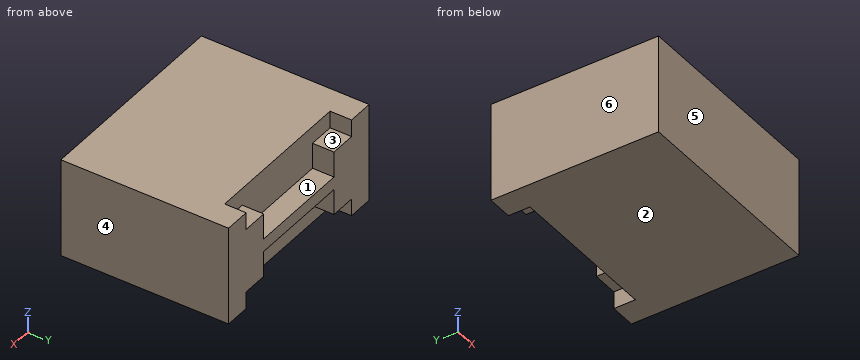
from build123d import *

# Parameters (mm, degrees)
SKETCH_1_W               = 240
SKETCH_1_H               = 195
EXTRUDE_1_DEPTH          = 57.5
CUT_EXTRUDE_1_DEPTH      = 165.962116863
CUT_EXTRUDE_1_DEPTH_BACK = 50
CUT_EXTRUDE_START        = -20
CUT_EXTRUDE_2_OUTLINE_W  = 30
CUT_EXTRUDE_2_OUTLINE_H  = 25
CUT_EXTRUDE_2_DEPTH      = 20


# Read off the part's stored shape, not the designer's step: 切除-拉伸2
with BuildPart() as part:
    # 草图1 → 凸台-拉伸1 (new body)
    with BuildSketch(Plane.XY):
        Rectangle(SKETCH_1_W, SKETCH_1_H)
    extrude(amount=EXTRUDE_1_DEPTH)

    # 草图2 → 切除-拉伸1 (cut, two sides: drawn at the far end of the back side and taken through both)
    with BuildSketch(Plane.XY.offset(57.5).offset(-CUT_EXTRUDE_1_DEPTH_BACK)):
        Polygon((-60, 638.254180389), (-60, 97.5), (-60, 72.5), (60, 72.5), (60, 97.5), (60, 638.254180389), (60, 1719.762541166), (-60, 1719.762541166), align=None)
    extrude(amount=CUT_EXTRUDE_1_DEPTH + CUT_EXTRUDE_1_DEPTH_BACK, mode=Mode.SUBTRACT)

    # 切除-拉伸2 outline → 切除-拉伸2 (cut)
    with BuildSketch(Plane.XY.offset(57.5).offset(CUT_EXTRUDE_START)):
        with Locations((-75, 85)):
            Rectangle(CUT_EXTRUDE_2_OUTLINE_W, CUT_EXTRUDE_2_OUTLINE_H)
    cut_extrude_2 = extrude(amount=CUT_EXTRUDE_2_DEPTH, mode=Mode.SUBTRACT)

    # 镜向1: 切除-拉伸2 across plane
    add(cut_extrude_2.mirror(Plane(origin=(0, 0, 0), x_dir=(0, 0, 1), z_dir=(1, 0, 0))), mode=Mode.SUBTRACT)

    # 镜向2: part across plane


with BuildPart() as part_1:
    add(part.part)
    add(part.part.mirror(Plane(origin=(0, 0, 0), x_dir=(1, 0, 0), z_dir=(0, 0, -1))))


solid = part_1.part
Geometry check sheet. Reference: the model listing, model coordinates, mm. Face numbers are marked on the shaded views. A direction names the side the tool comes from. Round coordinates to 2 decimals unless told otherwise and drop trailing zeros. Write each loop counter-clockwise with the first axis right and the second up, starting at its lowest first coordinate (ties: lowest second). Pieces come first, ordered by that corner, then holes.
Item 1: Mould release check, pull along X, two halves, no side actions. Record for the marked faces 3, 4, 5 and 6: +X half, -X half, draft (parallel to the pull), parting line (faces both ways), or undercut.
Determined:
face 3: undercut
face 4: +X half
face 5: draft
face 6: -X half
Item 2: Access from +Z, -Z, +X, -X, +Y, -Y to the whole of each face (thin tool, end or side, straight path). Record for the marked faces 1 and 2.
Determined:
face 1: +Z, +Y
face 2: -Z, +X, -X, +Y, -Y
Item 3: Section check A-A (z = 16.5). Record the boundary of the cut face in (x, y), plus the area to 3 significant figures.
Determined:
outline: (-120, -97.5) - (120, -97.5) - (120, 97.5) - (60, 97.5) - (60, 72.5) - (-60, 72.5) - (-60, 97.5) - (-120, 97.5) - close
area: 43,800 mm2
Item 4: Material ranges on line 1 along X through (y, z) = (85, -28); line 2 along Y through (x, z) = (63.5, -48); line 3 along Z through (x, y) = (37.5, 87), recorded low to high.
Determined:
line 1: x = -120 to -60, 60 to 120
line 2: y = -97.5 to 72.5
line 3: z = -7.5 to 7.5
Item 5: Go/stop test with flat-tipped pins: pin 1 Ø15 at (x, z) = (-43, 40.5) entering from +Y; pin 2 Ø7.5 at (x, y) = (69.5, 91) entering from +Z; pin 3 Ø7.5 at (x, y) = (1.5, 82) entering from +Z; pin 4 Ø4 at (x, z) = (54.5, -9) entering from +Y. Record where each tip stops, or that it passes through.
Determined:
pin 1: stops at y = 72.5
pin 2: stops at z = 37.5
pin 3: stops at z = 7.5
pin 4: stops at y = 97.5
Item 6: Section check B-B (x = 66). Record the boundary of the cut face in (y, z).
Determined:
outline: (-97.5, -57.5) - (72.5, -57.5) - (72.5, -37.5) - (97.5, -37.5) - (97.5, 37.5) - (72.5, 37.5) - (72.5, 57.5) - (-97.5, 57.5) - close
